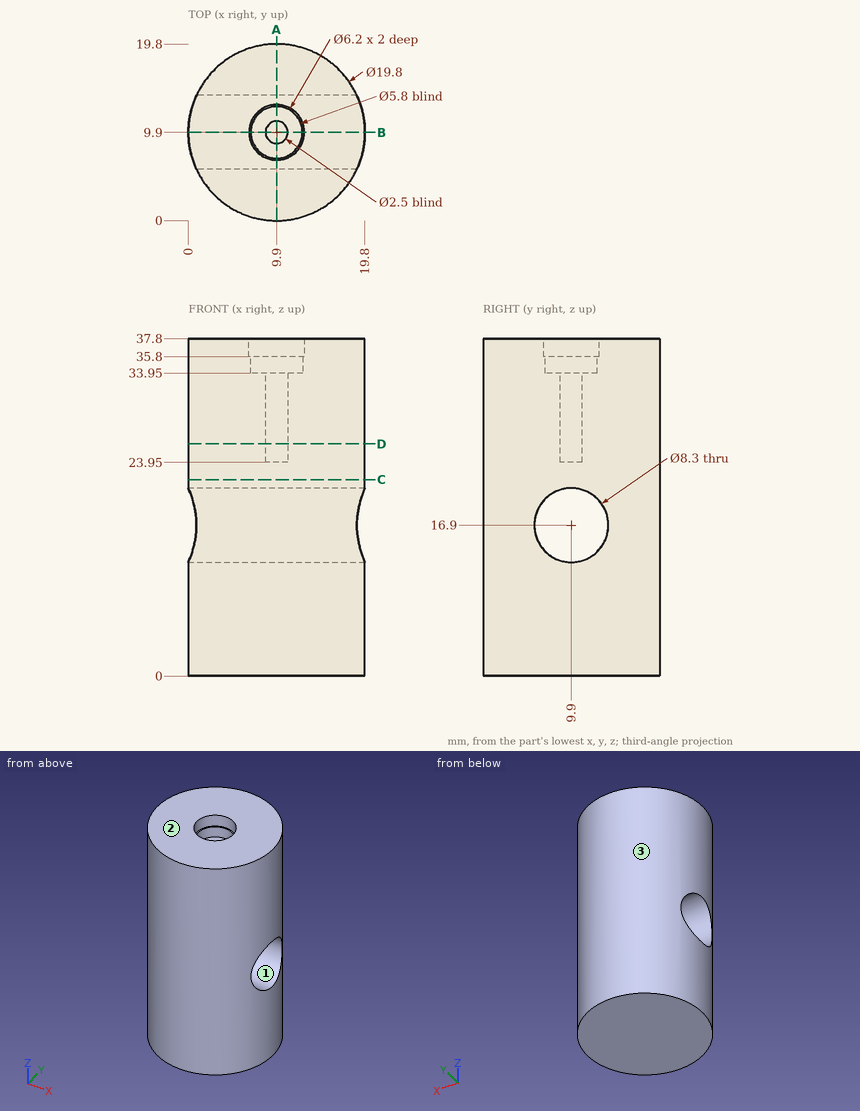
Here's the drawing with two shaded views (mm, measured from the low corner). I have some questions. Coordinates: 2 decimals unless noted, no trailing zeros. Write each loop counter-clockwise with the first axis right and the second up, starting at its lowest first coordinate (ties: lowest second). Pieces come first, ordered by that corner, then holes. Notation, with made-up numbers: (75.5, 38.25) - (82.5, 38.25) arc R22 ccw to (82.5, 54.25) - close; hole circle Ø10 at (-11, -37.75). An arc over 180 degrees is marked (long way). Return JSON: item names as keys, results as strings.
Q1. If we section it at B-B (y = 9.9): Please give me the cut outline in (x, z).
Computed values:
{"outline": "(0, 0) - (19.8, 0) - (19.8, 12.75) - (0, 12.75) - close; (0, 21.05) - (19.8, 21.05) - (19.8, 37.8) - (13, 37.8) - (13, 35.8) - (12.8, 35.8) - (12.8, 33.95) - (11.15, 33.95) - (11.15, 23.95) - (8.65, 23.95) - (8.65, 33.95) - (7, 33.95) - (7, 35.8) - (6.8, 35.8) - (6.8, 37.8) - (0, 37.8) - close"}
Q2. If we section it at A-A (x = 9.9): Please give me the cut outline in (y, z), then the cut area to 3 significant figures.
Computed values:
{"outline": "(0, 0) - (19.8, 0) - (19.8, 37.8) - (13, 37.8) - (13, 35.8) - (12.8, 35.8) - (12.8, 33.95) - (11.15, 33.95) - (11.15, 23.95) - (8.65, 23.95) - (8.65, 33.95) - (7, 33.95) - (7, 35.8) - (6.8, 35.8) - (6.8, 37.8) - (0, 37.8) - close; hole circle Ø8.3 at (9.9, 16.9)", "area": "646 mm2"}
Q3. Please list where these lines run through material, in increasing order: L1, parallel to Y at x = 9.9, z = 26.5; L2, parallel to Z at x = 5.75, y = 10; L3, parallel to Y at x = 9.9, z = 36.45. Write a range as from..to.
Computed values:
{"L1": "y = 0..8.65, 11.15..19.8", "L2": "z = 0..12.75, 21.05..37.8", "L3": "y = 0..6.8, 13..19.8"}
Q4. If we section it at D-D (z = 26): Please give me the cut outline in (x, y), then the cut area to 3 significant figures.
Computed values:
{"outline": "circle Ø19.8 at (9.9, 9.9); hole circle Ø2.5 at (9.9, 9.9)", "area": "303 mm2"}
Q5. If we section it at C-C (z = 22): Please give me the cut outline in (x, y), then the cut area to 3 significant figures.
Computed values:
{"outline": "circle Ø19.8 at (9.9, 9.9)", "area": "308 mm2"}
Q6. Thinking about a two-plate mould opening in Y: for the marked faces 1, 2 and 3, which applies, +Y half, -Y half, draft (parallel to the pull), parting line (faces both ways), or undercut?
Computed values:
{"face 1": "undercut", "face 2": "draft", "face 3": "parting line"}
Q7. I'm going to push flat-ended pins straight in: pin 1 Ø3 at (x, y) = (10, 11) entering from +Z; pin 2 Ø2 at (y, z) = (16.5, 7.5) entering from +X; pin 3 Ø5 at (y, z) = (7, 20) entering from -X; pin 4 Ø6.5 at (y, z) = (9.9, 16.9) entering from -X. Where does each tip first touch, or does it pass through?
Computed values:
{"pin 1": "stops at z = 33.95", "pin 2": "stops at x = 18.06", "pin 3": "stops at x = 0.02", "pin 4": "passes through"}
